Autodesk Inventor part; units mm, degrees
ref_plane "YZ Plane" through (0, 0, 0) normal (1, 0, 0) x (0, 1, 0)
ref_plane "XZ Plane" through (0, 0, 0) normal (0, 1, 0) x (-1, 0, 0)
ref_plane "XY Plane" through (0, 0, 0) normal (0, 0, 1) x (1, 0, 0)
sketch "Sketch1" plane through (0, 0, 0) normal (0, 0, 1) x (1, 0, 0)
  line L0 (-0.3861, 13.3644) -> (-0.3861, 12.1644)
  line L1 (0.8139, 10.5644) -> (0.8139, 13.3644)
  line L2 (2.7639, 27.7657) -> (2.7639, 5.268) construction
  line L3 (-5.7361, 13.3644) -> (-5.7361, 25.3644)
  line L4 (-2.7361, 28.3644) -> (2.7639, 28.3644)
  line L5 (2.7639, 26.8644) -> (-2.7361, 26.8644)
  line L6 (-4.2361, 25.3644) -> (-4.2361, 14.8644)
  line L7 (-4.2361, 14.8644) -> (2.7639, 14.8644)
  line L8 (-0.3861, 12.1644) -> (-0.8539, 11.8943)
  line L9 (-5.7361, 13.3644) -> (-0.3861, 13.3644)
  arc A0 (-2.7361, 28.3644) -> (-5.7361, 25.3644) centre (-2.7361, 25.3644) ccw
  arc A1 (-2.7361, 26.8644) -> (-4.2361, 25.3644) centre (-2.7361, 25.3644) ccw
  line L10 (-0.8539, 11.8943) -> (-0.0861, 10.5644)
  line L11 (-0.0861, 10.5644) -> (0.8139, 10.5644)
  line L12 (5.6139, 10.5644) -> (4.7139, 10.5644)
  line L13 (11.2639, 13.3644) -> (11.2639, 25.3644)
  arc A2 (11.2639, 25.3644) -> (8.2639, 28.3644) centre (8.2639, 25.3644) ccw
  line L14 (8.2639, 28.3644) -> (2.7639, 28.3644)
  line L15 (2.7639, 26.8644) -> (8.2639, 26.8644)
  arc A3 (9.7639, 25.3644) -> (8.2639, 26.8644) centre (8.2639, 25.3644) ccw
  line L16 (9.7639, 25.3644) -> (9.7639, 14.8644)
  line L17 (9.7639, 14.8644) -> (2.7639, 14.8644)
  line L18 (11.2639, 13.3644) -> (5.9139, 13.3644)
  line L19 (5.9139, 13.3644) -> (5.9139, 12.1644)
  line L20 (5.9139, 13.3644) -> (6.9559, 13.3644)
  line L21 (4.7139, 10.5644) -> (4.7139, 13.3644)
  line L22 (6.3817, 11.8943) -> (5.6139, 10.5644)
  line L23 (5.9139, 12.1644) -> (6.3817, 11.8943)
  line L24 (0.8139, 13.3644) -> (4.7139, 13.3644)
  line L25 (5.9139, 13.3644) -> (6.9559, 13.3644)
  point P0 (0, 0)
  dimension "d1" = 1.2
  dimension "d2" = 1.95
  dimension "d3" = 120
  dimension "d5" = 8.5
  dimension "d6" = 1.5
  dimension "d8" = 1.5
  dimension "d9" = 12
  dimension "d10" = 3
  dimension "d11" = 1.5
  dimension "d12" = 0.9
  dimension "d13" = 120
  dimension "d15" = 1.2
  dimension "d16" = 2.8
  dimension "d17" = 1.5
extrude "Extrusion1" add sketch "Sketch1" along normal blind 12
sketch "Sketch2" plane through (-2.7361, 28.3644, 0) normal (0, 1, 0) x (1, 0, 0)
  line L0 (0, -12) -> (11, -12)
  line L1 (11, 0) -> (0, 0)
  line L2 (0, 0) -> (0, -12)
  line L3 (1.5, 0) -> (3.1945, 0)
  line L4 (3.1945, 0) -> (9.5, -12)
  line L5 (7.8055, -12) -> (1.5, 0)
  point P0 (2.7361, 0)
  dimension "d20" = 1.5
  dimension "d21" = 1.5
  dimension "d22" = 1.5
extrude "Extrusion2" cut sketch "Sketch2" against normal up to next contours L5 L1 L4 L0
sketch "Sketch3" plane through (11.2639, 13.3644, 0) normal (1, 0, 0) x (0, 0, -1)
  line L0 (-12, 12) -> (-12, 0)
  line L1 (0, 0) -> (-12, 0)
  arc A0 (-7.75, 2.75) -> (-7.75, 1.25) centre (-7.75, 2) ccw
  arc A1 (-4.25, 1.25) -> (-4.25, 2.75) centre (-4.25, 2) ccw
  line L2 (-7.75, 2.75) -> (-4.25, 2.75)
  line L3 (-4.25, 1.25) -> (-7.75, 1.25)
  point P0 (0, -13.3644)
  dimension "d30" = 1.5
  dimension "d31" = 3.5
  dimension "d32" = 4.25
  dimension "d33" = 2
extrude "Extrusion3" cut sketch "Sketch3" against normal through all
properties part number "Cable V3"
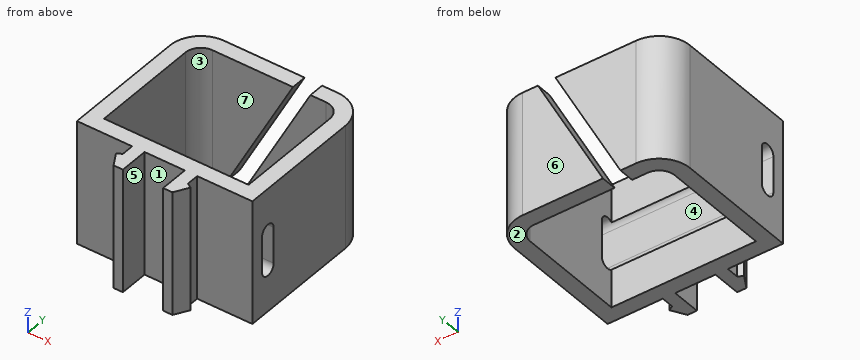
Here's how the part is built. I have some questions about the finished solid (model axes, mm). Face numbers are marked on the shaded views. A direction names the side the tool comes from. Give positions to 0.01 mm unless a question says otherwise; leave off trailing zeros. Write each loop counter-clockwise with the first axis right and the second up, starting at its lowest first coordinate (ties: lowest second). Pieces come first, ordered by that corner, then holes. Notation, with made-up numbers: M -11.5,-11 L 39.5,-11 A21 ccw 39.5,-2 Z; hole C -36.75,-40 d2. An arc over 180 degrees is marked long. Put each result on its own line as item: value. Start each with the question number.
Item 1: If we section it at D-D, the plane z = 9.5: Write out the boundary of the cut face in (x, y), then the cut area to 3 significant figures.
Item 2: If we section it at B-B, the plane z = 6.25: Count the separate pieces of the cut face and the enclosed holes in it, then the cut area to 3 significant figures.
Item 3: I need wall thicknesses on L1, parallel to Y at x = 0.5, z = 4.5; L2, parallel to Y at x = -1, z = 10.75; L3, parallel to X at y = 24.5, z = 9.75. Which ranges of each line are inside material? Lowest first, please. Write a range as from..to.
Item 4: On a 3-axis mill with a long thin cutter (end or side, diameter ignored), from which of +Z, -Z, +X, -X, +Y, -Y can I reach the whole of each face in a straight line? I mean the marked faces 1, 2 and 3. Say none if no direction works.
Item 5: If we section it at C-C, the plane x = 10: Write out the boundary of the cut face in (y, z).
Item 6: If we section it at A-A, the plane y = 16.5: Write out the boundary of the cut face in (x, z).
Item 7: Thinking about a two-plate mould opening in Y: for the marked faces 4, 5, 6 and 7, which applies, +Y half, -Y half, draft (parallel to the pull), parting line (faces both ways), or undercut?
Item 8: Will these pins go through, and if not, where does the flat tip stop? pin 1 (1.1 mm diameter, centred on x = 5, z = 9.5, fed in from +Y); pin 2 (4 mm diameter, centred on x = 6.5, y = 21, fed in from +Z); pin 3 (3 mm diameter, centred on y = 11.5, z = 4.5, fed in from +X); pin 4 (2.5 mm diameter, centred on x = -2.5, z = 5.5, fed in from -Y).
Values:
1. outline: M -5.74,13.36 L -0.39,13.36 L -0.39,12.16 L -0.85,11.89 L -0.09,10.56 L 0.81,10.56 L 0.81,13.36 L 4.71,13.36 L 4.71,10.56 L 5.61,10.56 L 6.38,11.89 L 5.91,12.16 L 5.91,13.36 L 11.26,13.36 L 11.26,25.36 A3 ccw 8.26,28.36 L 5.45,28.36 L 5.45,26.86 L 8.26,26.86 A1.5 cw 9.76,25.36 L 9.76,14.86 L -4.24,14.86 L -4.24,25.36 A1.5 cw -2.74,26.86 L 3.76,26.86 L 3.76,28.36 L -2.74,28.36 A3 ccw -5.74,25.36 Z
1. area: 88.6 mm²
2. separate pieces: 3
2. enclosed holes: 0
2. area: 80.6 mm²
3. L1: 10.56..14.61, 26.86..28.36
3. L2: 13.36..14.86, 26.86..28.36
3. L3: -5.74..-4.24, 9.76..11.26
4. face 1: +Z, -Z, -Y
4. face 2: -Z, +X, -X, +Y, -Y
4. face 3: +Z, -Z
5. outline: M 13.36,0 L 27.81,0 L 27.81,12 L 13.36,12 Z; hole M 14.61,4.25 A0.75 ccw 16.11,4.25 L 16.11,7.75 A0.75 ccw 14.61,7.75 Z
6. outline: M -5.74,0 L -4.24,0 L -4.24,12 L -5.74,12 Z; M 9.76,0 L 11.26,0 L 11.26,12 L 9.76,12 Z
7. face 4: undercut
7. face 5: draft
7. face 6: +Y half
7. face 7: undercut
8. pin 1: y = 28.36
8. pin 2: through
8. pin 3: x = 6.38
8. pin 4: y = 13.36
